from build123d import *
from build123d.topology import SkipClean

# Parameters (mm, degrees)
SKETCH14_R          = 4
SKETCH14_R_2        = 1.2
SKETCH14_R_3        = 5
BOSS_EXTRUDE1_DEPTH = 4
CUT_EXTRUDE1_START  = -2.5
SKETCH15_R          = 1.2
CUT_EXTRUDE1_DEPTH  = 1.5
CUT_EXTRUDE2_DEPTH  = 0.5
SKETCH17_R          = 1
CUT_EXTRUDE3_DEPTH  = 6
SKETCH18_R          = 2.25
CUT_EXTRUDE4_DEPTH  = 10


with BuildPart() as part:
    # Sketch14 → Boss-Extrude1 (new body)
    with BuildSketch(Plane.XY):
        with BuildLine():
            Line((30.133333333, 3.99777716), (0.166666667, 4.99722145))
            ThreePointArc((0.166666667, 4.99722145), (3.593976442, 3.476108936), (5, 0))
            ThreePointArc((5, 0), (3.593976442, -3.476108936), (0.166666667, -4.99722145))
            Line((0.166666667, -4.99722145), (30.133333333, -3.99777716))
            ThreePointArc((30.133333333, -3.99777716), (26, 0), (30.133333333, 3.99777716))
        make_face()
        with Locations((30, 0)):
            Circle(SKETCH14_R)
        with Locations((30, 0)):
            Circle(SKETCH14_R_2, mode=Mode.SUBTRACT)
        Circle(SKETCH14_R_3)
        Circle(SKETCH14_R_2, mode=Mode.SUBTRACT)
    extrude(amount=BOSS_EXTRUDE1_DEPTH)

    # Sketch15 → Cut-Extrude1 (cut)
    with BuildSketch(Plane.XY.offset(4).offset(CUT_EXTRUDE1_START)):
        with BuildLine():
            Line((16.121698113, 2.33951917), (0.363207547, 3.832829278))
            ThreePointArc((0.363207547, 3.832829278), (-3.85, 0), (0.363207547, -3.832829278))
            Line((0.363207547, -3.832829278), (16.121698113, -2.33951917))
            ThreePointArc((16.121698113, -2.33951917), (18.25, 0), (16.121698113, 2.33951917))
        make_face()
        Circle(SKETCH15_R, mode=Mode.SUBTRACT)
    extrude(amount=-CUT_EXTRUDE1_DEPTH, mode=Mode.SUBTRACT)

    # Sketch16 → Cut-Extrude2 (cut)
    with SkipClean():  # the faces are left unmerged after this step: merging them gives an invalid solid
        with BuildSketch(Plane(origin=(0, 0, 1.5), x_dir=(-1, 0, 0), z_dir=(0, 0, -1))):
            with BuildLine():
                ThreePointArc((-0.363207547, -3.832829278), (-3.85, 0), (-0.363207547, 3.832829278))
                Line((-0.363207547, 3.832829278), (-6, 3.298674112))
                Line((-6, 3.298674112), (-6, -3.298674112))
                Line((-6, -3.298674112), (-0.363207547, -3.832829278))
            make_face()
            with BuildLine():
                ThreePointArc((3.85, 0), (2.722361108, 2.722361108), (0, 3.85))
                Line((0, 3.85), (0, 1.2))
                ThreePointArc((0, 1.2), (0.848528137, 0.848528137), (1.2, 0))
                ThreePointArc((1.2, 0), (0.848528137, -0.848528137), (0, -1.2))
                Line((0, -1.2), (0, -3.85))
                ThreePointArc((0, -3.85), (2.722361108, -2.722361108), (3.85, 0))
            make_face()
            with BuildLine():
                Line((0, 1.2), (0, 3.85))
                ThreePointArc((0, 3.85), (-0.181806598, 3.845704924), (-0.363207547, 3.832829278))
                ThreePointArc((-0.363207547, 3.832829278), (-3.85, 0), (-0.363207547, -3.832829278))
                ThreePointArc((-0.363207547, -3.832829278), (-0.181806598, -3.845704924), (0, -3.85))
                Line((0, -3.85), (0, -1.2))
                ThreePointArc((0, -1.2), (-1.2, 0), (0, 1.2))
            make_face()
        extrude(amount=-CUT_EXTRUDE2_DEPTH, mode=Mode.SUBTRACT)

    # Sketch17 → Cut-Extrude3 (cut)
    with SkipClean():  # the faces are left unmerged after this step: merging them gives an invalid solid
        with BuildSketch(Plane(origin=(0, 0, 1.5), x_dir=(-1, 0, 0), z_dir=(0, 0, -1))):
            with Locations((-11.1, 0)):
                Circle(SKETCH17_R)
        extrude(amount=-CUT_EXTRUDE3_DEPTH, mode=Mode.SUBTRACT)

    # Sketch18 → Cut-Extrude4 (cut)
    with SkipClean():  # the faces are left unmerged after this step: merging them gives an invalid solid
        with BuildSketch(Plane.XY.offset(4)):
            Circle(SKETCH18_R)
        extrude(amount=-CUT_EXTRUDE4_DEPTH, mode=Mode.SUBTRACT)


solid = part.part
Work out the finished part from the listing and answer in its coordinate system (mm). A direction names the side the tool comes from. Give positions to 0.01 mm unless a question says otherwise; leave off trailing zeros. Loops run counter-clockwise (first coordinate to the right, second up) from the corner with the lowest first, then second, coordinate; pieces in that order, holes last. Notation, with made-up numbers: (64.25, -10) -> (106.25, -10) arc R33 cw to (106.25, 19) -> close; hole circle Ø6 at (10.5, 62). An arc over 180 degrees is marked (long way). Use a Markdown table: item, result. Add a question column.
1. For faces 4 (the flat face through (14, 0, 4)), 5 (the flat face through (2.24, 0.91, 2)), determine the directions among +Z, -Z, +X, -X, +Y, -Y from which every point of the face is accessible in a straight line to the end or side of a thin tool.
2. Determine the mould class of faces 1 (the cylindrical face through (34, 0, 2)), 2 (the flat face through (19, 0, 0)), 3 (the cylindrical face through (18.25, -0.05, 0.76)) for opening direction X: released by +X, released by -X, zero draft, split by the parting line, or undercut.
3. Flat-ended cylindrical pins translate along their axes: pin 1 Ø1 at (y, z) = (-1.5, 1.5) entering from +X; pin 2 Ø1.4 at (x, y) = (30, 0) entering from +Z; pin 3 Ø1.5 at (x, z) = (22, 1.5) entering from -Y; pin 4 Ø4 at (x, y) = (3, 0) entering from -Z. Find the tip coordinate at first contact, or state that the pin passes through.
4. Find the intervals of material crossed by probe 1 along Y at (x, z) = (30, 2.55); probe 2 along Y at (x, z) = (0, 3.15); probe 3 along Z at (x, y) = (15, 1.75), in increasing order.
5. Section A-A on z = 2.5 is taken. Determine the outline of the cut face in (x, y).
6. Section D-D on x = 30.5 is taken. Determine the outline of the cut face in (y, z), and give its area (3 significant figures).
7. Section B-B on z = 0.7 is taken. Determine the outline of the cut face in (x, y).
8. Section C-C on y = 1.75 is taken. Determine the outline of the cut face in (x, z), and give its area (3 significant figures).
Results below:
| question | item | result |
|---|---|---|
| 1 | face 4 | +Z, +X, -X, +Y, -Y |
| 1 | face 5 | -Z |
| 2 | face 1 | released by +X |
| 2 | face 2 | zero draft |
| 2 | face 3 | undercut |
| 3 | pin 1 | stops at x = 33.87 |
| 3 | pin 2 | passes through |
| 3 | pin 3 | stops at y = -4.29 |
| 3 | pin 4 | stops at z = 2 |
| 4 | probe 1 | y = -4 to -1.2, 1.2 to 4 |
| 4 | probe 2 | y = -5 to -2.25, 2.25 to 5 |
| 4 | probe 3 | z = 1.5 to 4 |
| 5 | outline | (0.17, -5) -> (30.13, -4) arc R4 ccw to (30.13, 4) -> (0.17, 5) arc R5 ccw (long way) to start; hole circle Ø4.5 at (0, 0); hole circle Ø2 at (11.1, 0); hole circle Ø2.4 at (30, 0) |
| 6 | outline | (-3.97, 0) -> (-1.09, 0) -> (-1.09, 4) -> (-3.97, 4) -> close; (1.09, 0) -> (3.97, 0) -> (3.97, 4) -> (1.09, 4) -> close |
| 6 | area | 23.0 mm^2 |
| 7 | outline | (0.17, -5) -> (30.13, -4) arc R4 ccw to (30.13, 4) -> (0.17, 5) arc R5 ccw (long way) to start; hole (0.36, -3.83) -> (16.12, -2.34) arc R2.35 ccw to (16.12, 2.34) -> (0.36, 3.83) arc R3.85 ccw (long way) to start; hole circle Ø2.4 at (30, 0) |
| 8 | outline | (-4.68, 0) -> (-3.43, 0) -> (-3.43, 2) -> (-1.41, 2) -> (-1.41, 4) -> (-4.68, 4) -> close; (1.41, 2) -> (6, 2) -> (6, 1.5) -> (17.47, 1.5) -> (17.47, 0) -> (33.6, 0) -> (33.6, 4) -> (1.41, 4) -> close |
| 8 | area | 111 mm^2 |
